Source: CAD feature listing. Evaluate the final solid. Frame: model axes, mm. A direction names the side the tool comes from. Give positions to 0.01 mm unless a question says otherwise; leave off trailing zeros. Order: outer loops, then holes, each group sorted by start corner. A loop starts at its lowest first (then second) coordinate and runs counter-clockwise, first axis right, second up. Notation, with made-up numbers: M -2,6 L 38,6 A7 ccw 38,11 Z; hole C 89,-12 d11. An arc over 180 degrees is marked long. Answer in a Markdown table with one row per item. Add a question column.
(1) Pin query (flat end, axial travel): P1, Ø2, axis at x = 0, z = 15, coming from the +Y side; P2, Ø2, axis at y = -28, z = -6, coming from the -X side; P3, Ø2, axis at x = 4.5, y = -18.5, coming from the -Z side. Return the tip coordinate at first contact, or that it passes through.
(2) Section query A-A, the plane z = 0. Return loops of the section in (x, y), plus the area to 3 significant figures.
(3) Section query D-D, the plane z = -7. Return loops of the section in (x, y).
(4) Material intervals for line 1 along Z through (x, y) = (0, 4.5); line 2 along Z through (x, y) = (0, 1.5); line 3 along X through (y, z) = (3, -15), sorted ascending.
(5) Set-up query: faces 1 (the face through (0, -42, 0)), 2 (the face through (-7, -2, 0)). Return all of +Z, -Z, +X, -X, +Y, -Y with unobstructed straight access to the full face (end or side cutting, diameter ignored); none if empty.
(6) Mould query, pull axis Z, two halves, no side actions, for faces 3 (the face through (0, 1, 19)), 4 (the face through (0.65, 3.06, -16.57)), 5 (the face through (-13.466, 5.745, -0.14)). Classes: pulls with the +Z half, pulls with the -Z half, needs draft (parallel to the pull), parting line crosses it, or undercut.
(7) Section query C-C, the plane y = -20. Return loops of the section in (x, z), plus the area to 3 significant figures.
(8) Section query B-B, the plane y = 4.5. Count the separate pieces of the cut face and the enclosed holes in it, plus the area to 3 significant figures.
Autodesk Inventor part; units mm, degrees
ref_plane "YZ Plane" through (0, 0, 0) normal (1, 0, 0) x (0, 1, 0)
ref_plane "XZ Plane" through (0, 0, 0) normal (0, 1, 0) x (-1, 0, 0)
ref_plane "XY Plane" through (0, 0, 0) normal (0, 0, 1) x (1, 0, 0)
sketch "Sketch1" plane through (0, 0, 0) normal (0, 0, 1) x (1, 0, 0)
  arc A0 (-12.941, 7.7037) -> (12.941, 7.7037) centre (0, 56) ccw
  arc A1 (-14.4939, 1.9082) -> (14.4939, 1.9082) centre (0, 56) ccw
  line L0 (-14.4939, 1.9082) -> (-12.941, 7.7037)
  line L1 (14.4939, 1.9082) -> (12.941, 7.7037)
  line L2 (0, -11.2) -> (0, 67.2) construction
  point P0 (0, 0)
  dimension "d0" = 6
  dimension "d1" = 50
  dimension "d2" = 30
extrude "Extrusion1" add sketch "Sketch1" along normal mid plane 40
sketch "Sketch2" plane through (0, 0, 0) normal (0, 1, 0) x (-1, 0, 0)
  point P0 (0, 0)
  point P1 (0, -15)
  point P2 (0, 15)
  dimension "d5" = 15
  dimension "d6" = 15
hole "Hole1" at (0, 0, -15) at (0, 0, 15) direction (0, 1, 0) diameter 3.4 end through all
sketch "Sketch4" plane through (0, 0, 0) normal (0, 1, 0) x (-1, 0, 0)
  circle A0 centre (0, 0) radius 10
  dimension "d20" = 20
extrude "Extrusion3" add sketch "Sketch4" along normal up to surface
extrude "Extrusion4" add sketch "Sketch4" against normal blind 2
fillet "Fillet2" radius 10 4 edges at (-13.7174, 4.8059, -20) (13.7174, 4.8059, -20) (13.7174, 4.8059, 20) (-13.7174, 4.8059, 20)
sketch "Sketch6" plane through (0, -2, 0) normal (0, -1, 0) x (1, 0, 0)
  circle A0 centre (0, 0) radius 6
  dimension "d27" = 12
extrude "Extrusion5" add sketch "Sketch6" along normal blind 40
chamfer "Chamfer1" distance 2 angle 45 4 edges at (14.4939, 1.9082, 0) (0, 0, -20) (-14.4939, 1.9082, 0) (0, 0, 20)
properties part number "Mount_A"
Values follow:
| question | item | result |
|---|---|---|
| 1 | P1 | passes through |
| 1 | P2 | stops at x = -3.32 |
| 1 | P3 | stops at z = -4.87 |
| 2 | outline | M -13.98,3.84 L -12.55,1.43 A56 ccw -10,0.9 L -10,-2 L -6,-2 L -6,-42 L 6,-42 L 6,-2 L 10,-2 L 10,0.9 A56 ccw 12.55,1.43 L 13.98,3.84 L 12.94,7.7 A50 cw -12.94,7.7 Z |
| 2 | area | 688 mm² |
| 3 | outline | M -13.98,3.84 L -12.55,1.43 A56 ccw -7.14,0.46 L -7.14,-2 L 7.14,-2 L 7.14,0.46 A56 ccw 12.55,1.43 L 13.98,3.84 L 12.94,7.7 A50 cw -12.94,7.7 Z |
| 4 | line 1 | z = -20 to -16.7, -13.3 to 13.3, 16.7 to 20 |
| 4 | line 2 | z = -19.5 to -16.7, -13.3 to 13.3, 16.7 to 19.5 |
| 4 | line 3 | x = -12.31 to -1.7, 1.7 to 12.31 |
| 5 | face 1 | +Z, -Z, +X, -X, -Y |
| 5 | face 2 | -Y |
| 6 | face 3 | pulls with the +Z half |
| 6 | face 4 | undercut |
| 6 | face 5 | needs draft |
| 7 | outline | C 0,0 d12 |
| 7 | area | 113 mm² |
| 8 | separate pieces | 1 |
| 8 | enclosed holes | 2 |
| 8 | area | 997 mm² |
